Source: three-view drawing plus pictorial views. Frame: mm from the lowest corner of the part. A direction names the side the tool comes from. Coordinates: 2 decimals unless noted, no trailing zeros. Write each loop counter-clockwise with the first axis right and the second up, starting at its lowest first coordinate (ties: lowest second). Pieces come first, ordered by that corner, then holes. Notation, with made-up numbers: M -14.75,23 L -4.75,23 A32 cw -4.75,56 Z; hole C 3,-39 d4. An arc over 180 degrees is marked long. Use CSV: the item, a comma, the result in double quotes.
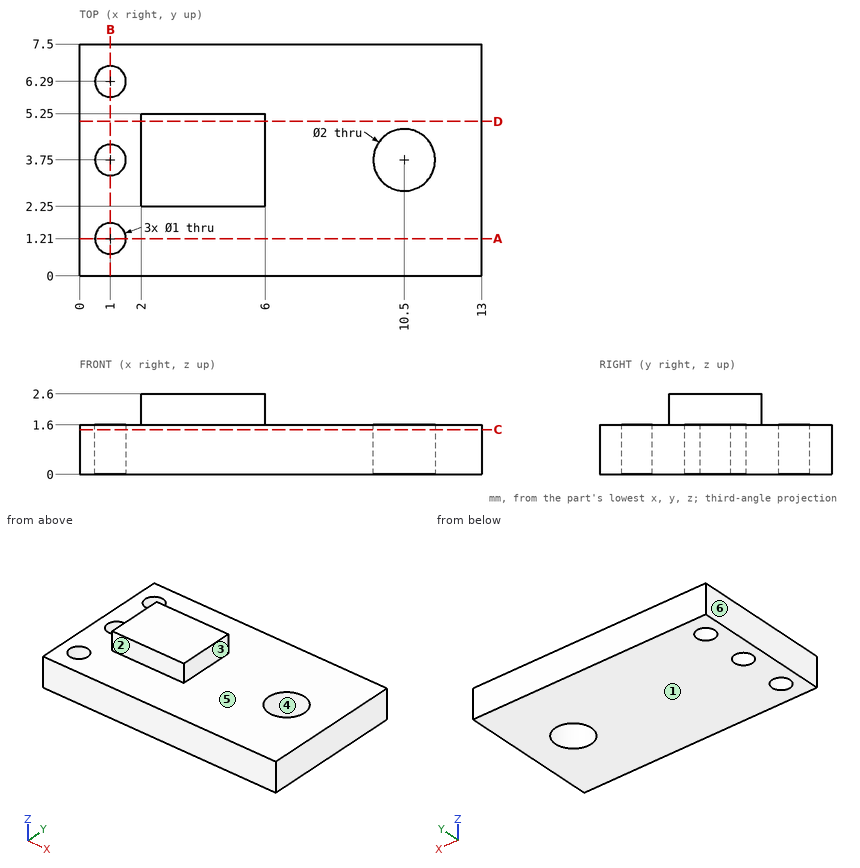
1. Access query for the marked faces 1 and 2. Directions: +Z, -Z, +X, -X, +Y, -Y. A direction counts if a zero-diameter tool reaches every point of the face in a straight line with its end or side. Return the directions, or none.
Resolved:
face 1,"-Z, +X, -X, +Y, -Y"
face 2,"+Z, +X, -X, -Y"
2. Section A-A (y = 1.21). Return loops of the section in (x, z).
Resolved:
outline,"M 0,0 L 0.5,0 L 0.5,1.6 L 0,1.6 Z; M 1.5,0 L 13,0 L 13,1.6 L 1.5,1.6 Z"
3. Section B-B (x = 1). Return loops of the section in (y, z).
Resolved:
outline,"M 0,0 L 0.71,0 L 0.71,1.6 L 0,1.6 Z; M 1.71,0 L 3.25,0 L 3.25,1.6 L 1.71,1.6 Z; M 4.25,0 L 5.79,0 L 5.79,1.6 L 4.25,1.6 Z; M 6.79,0 L 7.5,0 L 7.5,1.6 L 6.79,1.6 Z"
4. Mould query, pull axis X, two halves, no side actions, for the marked faces 3, 4, 5 and 6. Classes: pulls with the +X half, pulls with the -X half, needs draft (parallel to the pull), parting line crosses it, or undercut.
Resolved:
face 3,"pulls with the +X half"
face 4,"undercut"
face 5,"needs draft"
face 6,"pulls with the -X half"
5. Contact query for flat-ended pins moving along their axis: pin 1 Ø3 at (x, y) = (11, 2) entering from +Z; pin 2 Ø0.5 at (y, z) = (4, 2) entering from +X. Output: stop coordinate, or through.
Resolved:
pin 1,"stops at z = 1.6"
pin 2,"stops at x = 6"
6. Section C-C (z = 1.45). Return loops of the section in (x, y), then the cut area to 3 significant figures.
Resolved:
outline,"M 0,0 L 13,0 L 13,7.5 L 0,7.5 Z; hole C 1,1.21 d1; hole C 1,3.75 d1; hole C 1,6.29 d1; hole C 10.5,3.75 d2"
area,"92.0 mm^2"
7. Section D-D (y = 5). Return loops of the section in (x, z), then the cut area to 3 significant figures.
Resolved:
outline,"M 0,0 L 13,0 L 13,1.6 L 6,1.6 L 6,2.6 L 2,2.6 L 2,1.6 L 0,1.6 Z"
area,"24.8 mm^2"
8. Material intervals for line 1 (Y direction, x = 1, z = 0.55); line 2 (Y direction, x = 10.5, z = 0.65); line 3 (Z direction, x = 8.75, y = 6.25), sorted ascending. Write a range as [from, to].
Resolved:
line 1,"y = [0, 0.71], [1.71, 3.25], [4.25, 5.79], [6.79, 7.5]"
line 2,"y = [0, 2.75], [4.75, 7.5]"
line 3,"z = [0, 1.6]"
